The listing builds one solid part. Answer for the finished solid, in the listing's coordinates (mm). Face numbers are marked on the shaded views. A direction names the side the tool comes from. Coordinates: 2 decimals unless noted, no trailing zeros. Loops run counter-clockwise (first coordinate to the right, second up) from the corner with the lowest first, then second, coordinate; pieces in that order, holes last. Notation, with made-up numbers: (-39, 88.25) - (7, 88.25) arc R23 cw to (7, 125.25) - close; hole circle Ø8 at (64.25, -8). An arc over 180 degrees is marked (long way). One line per question, with ' | ' between items.
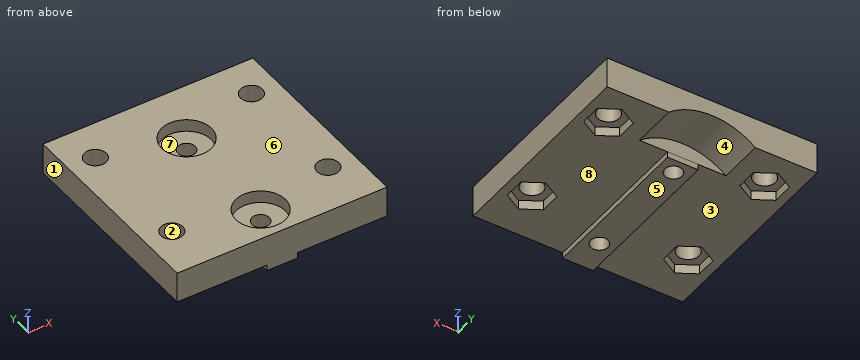
Autodesk Inventor part; units mm, degrees
ref_plane "YZ Plane" through (0, 0, 0) normal (1, 0, 0) x (0, 1, 0)
ref_plane "XZ Plane" through (0, 0, 0) normal (0, 1, 0) x (-1, 0, 0)
ref_plane "XY Plane" through (0, 0, 0) normal (0, 0, 1) x (1, 0, 0)
ref_plane "Work Plane7" through (21.5, 42.1122, 7.5565) normal (0, 0, -1) x (0, 1, 0)
sketch "Sketch4" plane through (21.5, 42.1122, 7.5565) normal (0, 0, -1) x (0, 1, 0)
  line L0 (-42.1122, -17.69) -> (-42.1122, -25.31) construction
  line L1 (0, 0) -> (0, -43) construction
  line L2 (-528, -43) -> (0, -43) construction
  line L3 (-528, 0) -> (0, 0) construction
  line L4 (-42.1122, -43) -> (0, -43)
  line L5 (0, -43) -> (0, 0)
  line L6 (0, 0) -> (-42.1122, 0)
  line L7 (-42.1122, 0) -> (-42.1122, -43)
  circle A0 centre (-8, -5.5) radius 2
  circle A1 centre (-32, -5.5) radius 2
  circle A2 centre (-8, -37.5) radius 2
  circle A3 centre (-32, -37.5) radius 2
  circle A4 centre (-8, -37.5) radius 2.2479
  circle A5 centre (-8, -5.5) radius 2.2479
  circle A6 centre (-32, -37.5) radius 2.2479
  point P0 (-42.1122, -21.5)
  dimension "d41" = 4.4958
  dimension "d42" = 4.4958
  dimension "d43" = 4.4958
extrude "Extrusion4" add sketch "Sketch4" along normal blind 6.35 contours L7 L6 L5 L4 | A4 | A5 | A6
ref_plane "Work Plane6" through (0, 0, 0) normal (0, 0, 1) x (1, 0, 0)
sketch "Sketch5" plane through (0, 0, 0) normal (0, 0, 1) x (1, 0, 0)
  line L0 (3.1132, 0) -> (3.1132, 33.02) construction
  line L1 (-3.1132, 0) -> (-3.1132, 33.02) construction
  line L2 (3.14, 32.92) -> (-3.14, 32.92) construction
  line L3 (-21.5, 0) -> (21.5, 0) construction
  line L4 (3.1132, 0) -> (-3.14, 0)
  line L5 (-3.14, 0) -> (-3.14, 32.92)
  line L6 (-3.14, 32.92) -> (3.1132, 32.92)
  line L7 (3.1132, 32.92) -> (3.1132, 0)
  arc A0 (-0.0115, 8.4836) -> (1.2335, 7.976) centre (0, 6.731) ccw construction
  spline S0 degree 3 poles (-3.9963, 27.1983) (-3.9282, 27.0439) (-3.8705, 26.8672) (-3.7787, 26.4733) (-3.747, 26.2579) (-3.7229, 25.8912) (-3.7161, 25.6578) (-3.7657, 25.2017) (-3.8042, 25.0235) (-3.9064, 24.7384) (-3.9674, 24.6297) (-4.0735, 24.5156) (-4.1125, 24.4855) (-4.225, 24.4328) (-4.3003, 24.4339) (-4.4555, 24.5079) (-4.5339, 24.5853) (-4.6625, 24.7855) (-4.7303, 24.9172) (-4.8354, 25.2648) (-4.8698, 25.4348) (-4.9129, 25.8035) (-4.9196, 25.9997) (-4.906, 26.2838) (-4.8978, 26.3737) (-4.8628, 26.6198) (-4.8272, 26.7652) (-4.7302, 27.0244) (-4.6681, 27.1326) (-4.5976, 27.2088) knots 0.000001 0.000001 0.000001 0.000001 0.061283 0.061283 0.126502 0.126502 0.171802 0.171802 0.206523 0.206523 0.238722 0.238722 0.255636 0.255636 0.285543 0.285543 0.317605 0.317605 0.342807 0.342807 0.362438 0.362438 0.383231 0.383231 0.393319 0.393319 0.411548 0.411548 0.431083 0.431083 0.431083 0.431083 construction
  circle A1 centre (0, 6.731) radius 1.778 construction
  circle A2 centre (-0.0134, 32.92) radius 1.778 construction
  point P0 (0, 0)
  dimension "d10" = 3.556
  dimension "d11" = 3.556
extrude "Extrusion5" add sketch "Sketch5" along normal up to surface (1.2065 mm away)
sketch "Sketch6" plane through (21.5, 42.1122, 7.5565) normal (0, 0, 1) x (1, 0, 0)
  arc A0 (-21.5115, -33.6287) -> (-20.2665, -34.1362) centre (-21.5, -35.3812) ccw construction
  arc A1 (-21.5115, -10.3793) -> (-20.2665, -10.8868) centre (-21.5, -12.1318) ccw construction
  point P0 (-21.5, -42.1122)
hole "Hole2" at (0, 6.731, 7.5565) at (0, 29.9804, 7.5565) direction (0, 0, -1) diameter 3.556 end through all
ref_plane "Work Plane8" through (21.5, 42.1122, 7.5565) normal (0, 0, 1) x (1, 0, 0)
sketch "Sketch7" plane through (21.5, 42.1122, 7.5565) normal (0, 0, 1) x (1, 0, 0)
  circle A0 centre (-21.5, -12.1318) radius 1.778
  circle A1 centre (-21.5, -12.1318) radius 5.08
  circle A2 centre (-21.5, -35.3812) radius 1.778
  circle A3 centre (-21.5, -35.3812) radius 5.08
  point P0 (-21.5, -42.1122)
  dimension "d28" = 10.16
  dimension "d29" = 10.16
extrude "Extrusion6" cut sketch "Sketch7" against normal blind 2.54
sketch "Sketch8" plane through (-21.5, 42.1122, 7.5565) normal (0, 1, 0) x (1, 0, 0)
  circle A0 centre (21.5, 17.145) radius 3.24 construction
  arc A1 (12.6327, 6.35) -> (30.3673, 6.35) centre (21.5, 17.145) ccw
  line L0 (0, 6.35) -> (43, 6.35)
  line L1 (12.6327, 6.35) -> (30.3673, 6.35)
  point P0 (21.5, 7.5565)
  dimension "d32" = 27.94
extrude "Extrusion7" cut sketch "Sketch8" against normal blind 9.1948
sketch "Sketch9" plane through (21.5, 42.1122, 1.2065) normal (0, 0, -1) x (-1, 0, 0)
  circle A0 centre (37.5, -8) radius 2 construction
  circle A1 centre (37.5, -8) radius 4.2545 construction
  circle A2 centre (37.5, -32) radius 2 construction
  circle A3 centre (37.5, -32) radius 4.2545 construction
  circle A4 centre (5.5, -8) radius 2 construction
  circle A5 centre (5.5, -8) radius 4.2545 construction
  circle A6 centre (5.5, -32) radius 2 construction
  circle A7 centre (5.5, -32) radius 4.2545 construction
  line L0 (5.5, -12.2545) -> (1.8155, -10.1272)
  line L1 (1.8155, -10.1272) -> (1.8155, -5.8727)
  line L2 (1.8155, -5.8727) -> (5.5, -3.7455)
  line L3 (5.5, -3.7455) -> (9.1845, -5.8727)
  line L4 (9.1845, -5.8727) -> (9.1845, -10.1272)
  line L5 (9.1845, -10.1272) -> (5.5, -12.2545)
  line L6 (5.5, -36.2545) -> (1.8155, -34.1272)
  line L7 (1.8155, -34.1272) -> (1.8155, -29.8727)
  line L8 (1.8155, -29.8727) -> (5.5, -27.7455)
  line L9 (5.5, -27.7455) -> (9.1845, -29.8727)
  line L10 (9.1845, -29.8727) -> (9.1845, -34.1272)
  line L11 (9.1845, -34.1272) -> (5.5, -36.2545)
  line L12 (37.5, -12.2545) -> (33.8155, -10.1272)
  line L13 (33.8155, -10.1272) -> (33.8155, -5.8727)
  line L14 (33.8155, -5.8727) -> (37.5, -3.7455)
  line L15 (37.5, -3.7455) -> (41.1845, -5.8727)
  line L16 (41.1845, -5.8727) -> (41.1845, -10.1272)
  line L17 (41.1845, -10.1272) -> (37.5, -12.2545)
  line L18 (37.5, -36.2545) -> (33.8155, -34.1272)
  line L19 (33.8155, -34.1272) -> (33.8155, -29.8727)
  line L20 (33.8155, -29.8727) -> (37.5, -27.7455)
  line L21 (37.5, -27.7455) -> (41.1845, -29.8727)
  line L22 (41.1845, -29.8727) -> (41.1845, -34.1272)
  line L23 (41.1845, -34.1272) -> (37.5, -36.2545)
  point P0 (21.5, -42.1122)
  dimension "d35" = 8.509
  dimension "d36" = 8.509
  dimension "d37" = 8.509
  dimension "d38" = 8.509
extrude "Extrusion8" cut sketch "Sketch9" against normal blind 1.905
sketch "Sketch10" plane through (21.5, 42.1122, 7.5565) normal (0, 0, 1) x (1, 0, 0)
  circle A0 centre (-37.5, -32) radius 2
  circle A1 centre (-37.5, -32) radius 2.2479
  circle A2 centre (-5.5, -32) radius 2
  circle A3 centre (-5.5, -32) radius 2.2479
  circle A4 centre (-37.5, -8) radius 2
  circle A5 centre (-37.5, -8) radius 2.2479
  circle A6 centre (-5.5, -8) radius 2
  circle A7 centre (-5.5, -8) radius 2.2479
  point P0 (-21.5, -42.1122)
  dimension "d44" = 4.4958
  dimension "d45" = 4.4958
  dimension "d46" = 4.4958
  dimension "d47" = 4.4958
hole "Hole3" at (-16, 34.1122, 7.5565) at (-16, 10.1122, 7.5565) at (16, 10.1122, 7.5565) at (16, 34.1122, 7.5565) direction (0, 0, -1) diameter 4.4958 end through all
properties part number "LeadScrewNutCouplerForTrussHeadScrew"
Item 1: Find section D-D, the plane x = -11.5. Write down the section's boundary in (y, z), plus the area to 3 significant figures.
Taken from the geometry:
outline: (0, 1.21) - (42.11, 1.21) - (42.11, 7.56) - (0, 7.56) - close | area: 267 mm2
Item 2: Find section C-C, the plane y = 37. Write down the section's boundary in (x, z).
Taken from the geometry:
outline: (-21.5, 1.21) - (-18.37, 1.21) - (-18.37, 3.11) - (-13.63, 3.11) - (-13.63, 1.21) - (-8.87, 1.21) arc R13.97 cw to (8.87, 1.21) - (13.63, 1.21) - (13.63, 3.11) - (18.37, 3.11) - (18.37, 1.21) - (21.5, 1.21) - (21.5, 7.56) - (-21.5, 7.56) - close
Item 3: Find section B-B, the plane z = 6.25. Write down the section's boundary in (x, y).
Taken from the geometry:
outline: (-21.5, 0) - (21.5, 0) - (21.5, 42.11) - (-21.5, 42.11) - close; hole circle Ø4.5 at (-16, 10.11); hole circle Ø4.5 at (-16, 34.11); hole circle Ø10.16 at (0, 6.73); hole circle Ø10.16 at (0, 29.98); hole circle Ø4.5 at (16, 10.11); hole circle Ø4.5 at (16, 34.11)
Item 4: The mould has two halves that part along X. Classify the marked faces 1, 2 and 3: pulls with the +X half, pulls with the -X half, needs draft (parallel to the pull), parting line crosses it, or undercut.
Taken from the geometry:
face 1: pulls with the -X half | face 2: undercut | face 3: needs draft
Item 5: Each of these flat-tipped pins is pushed along its axis until it touches: pin 1 Ø5 at (x, y) = (-10.5, 31.5) entering from -Z; pin 2 Ø6 at (x, y) = (-16, 10.11) entering from -Z; pin 3 Ø1.3 at (y, z) = (8.5, 0.5) entering from +X. Where does it stop, or does it pass through?
Taken from the geometry:
pin 1: stops at z = 1.21 | pin 2: stops at z = 3.11 | pin 3: stops at x = 3.11
Item 6: Find section A-A, the plane x = 0. State how many separate pieces and enclosed holes the cut face has, plus the area to 3 significant figures.
Taken from the geometry:
separate pieces: 3 | enclosed holes: 0 | area: 191 mm2
Item 7: Find the intervals of material crossed by line 1 (Y direction, x = 16, z = 4.15); line 2 (Y direction, x = 0, z = 2.4); line 3 (X direction, y = 13.5, z = 3), in increasing order. Write a range as [from, to].
Taken from the geometry:
line 1: y = [0, 7.86], [12.36, 31.86], [36.36, 42.11] | line 2: y = [0, 4.95], [8.51, 28.2], [31.76, 32.92] | line 3: x = [-21.5, -17.5], [-14.5, 14.5], [17.5, 21.5]
Item 8: Which of the six approach directions +Z, -Z, +X, -X, +Y, -Y give full straight-line access (tool end or side, diameter ignored) to the marked faces 4, 5, 6, 7 and 8?
Taken from the geometry:
face 4: -Z, +Y | face 5: -Z, +X, -X, +Y, -Y | face 6: +Z, +X, -X, +Y, -Y | face 7: +Z | face 8: -Z, +X, +Y, -Y
